```python
from build123d import *

# Parameters (mm, degrees)
MODEL_R                 = 1.5
MODEL_R_2               = 4.000000302
SALIENTE_EXTRUIR1_DEPTH = 3


with BuildPart() as part:
    # Model → Saliente-Extruir1 (new body)
    with BuildSketch(Plane.XY):
        with BuildLine():
            Line((33.092598, 34.66167), (33.092598, -17.33833))
            Line((33.092598, -17.33833), (-2.449857, -8.810201))
            ThreePointArc((-2.449857, -8.810201), (-10.360174953, -0.307858771), (-5.597443, 10.283616))
            Line((-5.597443, 10.283616), (33.092598, 34.66167))
        make_face()
        with Locations((7.5, 1.4)):
            Circle(MODEL_R, mode=Mode.SUBTRACT)
        with Locations((-7.5, 1.4)):
            Circle(MODEL_R, mode=Mode.SUBTRACT)
        with Locations((-3.02e-07, 1.399999887)):
            Circle(MODEL_R_2, mode=Mode.SUBTRACT)
    extrude(amount=SALIENTE_EXTRUIR1_DEPTH)


solid = part.part
```
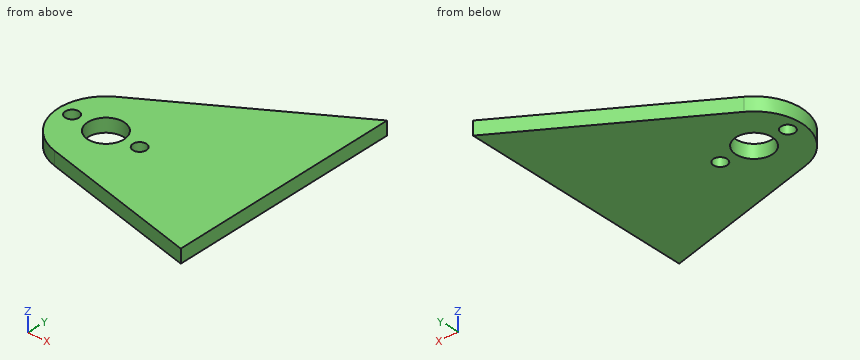
CAD build for the part. Positions are in the model's coordinates, mm. Give positions to 0.01 mm unless a question says otherwise; leave off trailing zeros. Write each loop counter-clockwise with the first axis right and the second up, starting at its lowest first coordinate (ties: lowest second). Pieces come first, ordered by that corner, then holes. Notation, with made-up numbers: (1, 57) -> (25, 57) arc R17 cw to (25, 87) -> close; hole circle Ø1 at (-32, 83). An arc over 180 degrees is marked (long way). Write each question's results on one line, items separated by ' | '.
1. Cut at D-D, the plane x = 7.5. Write the cut outline in (y, z).
Geometry check:
outline: (-11.2, 0) -> (-0.1, 0) -> (-0.1, 3) -> (-11.2, 3) -> close; (2.9, 0) -> (18.54, 0) -> (18.54, 3) -> (2.9, 3) -> close
2. Wall check: probe 1 along Y at (x, z) = (1, 0.2); probe 2 along Y at (x, z) = (0, 1.05); probe 3 along Y at (x, z) = (18.5, 2.2). Give the ranges that are in metal, low to high. Write a range as [from, to].
Geometry check:
probe 1: [-9.64, -2.47], [5.27, 14.44] | probe 2: [-9.4, -2.6], [5.4, 13.81] | probe 3: [-13.84, 25.47]
3. Cut at A-A, the plane y = 1.4. Write the cut outline in (x, z), then the cut area to 3 significant figures.
Geometry check:
outline: (-10.5, 0) -> (-9, 0) -> (-9, 3) -> (-10.5, 3) -> close; (-6, 0) -> (-4, 0) -> (-4, 3) -> (-6, 3) -> close; (4, 0) -> (6, 0) -> (6, 3) -> (4, 3) -> close; (9, 0) -> (33.09, 0) -> (33.09, 3) -> (9, 3) -> close | area: 88.8 mm²
4. Cut at C-C, the plane x = -7.5. Write the cut outline in (y, z), then the cut area to 3 significant figures.
Geometry check:
outline: (-5.95, 0) -> (-0.1, 0) -> (-0.1, 3) -> (-5.95, 3) -> close; (2.9, 0) -> (8.75, 0) -> (8.75, 3) -> (2.9, 3) -> close | area: 35.1 mm²
5. Cut at B-B, the plane z = 2. Write the cut outline in (x, y), then the cut area to 3 significant figures.
Geometry check:
outline: (-5.6, 10.28) arc R10.5 ccw to (-2.45, -8.81) -> (33.09, -17.34) -> (33.09, 34.66) -> close; hole circle Ø3 at (-7.5, 1.4); hole circle Ø8 at (0, 1.4); hole circle Ø3 at (7.5, 1.4) | area: 1,360 mm²
